Autodesk Inventor part; units mm, degrees
ref_plane "YZ Plane" through (0, 0, 0) normal (1, 0, 0) x (0, 1, 0)
ref_plane "XZ Plane" through (0, 0, 0) normal (0, 1, 0) x (-1, 0, 0)
ref_plane "XY Plane" through (0, 0, 0) normal (0, 0, 1) x (1, 0, 0)
sketch "Sketch1" plane through (0, 0, 0) normal (0, 0, 1) x (1, 0, 0)
  line L0 (-133.35, -63.5) -> (133.35, -63.5)
  line L1 (133.35, -63.5) -> (133.35, 63.5)
  line L2 (133.35, 63.5) -> (-133.35, 63.5)
  line L3 (-133.35, 63.5) -> (-133.35, -63.5)
  line L4 (-133.35, -63.5) -> (133.35, 63.5) construction
  line L5 (133.35, -63.5) -> (-133.35, 63.5) construction
  line L6 (0, 88.9) -> (0, -88.9) construction
  circle A0 centre (0, 47.625) radius 6.35
  circle A1 centre (-88.9, -47.625) radius 6.35
  circle A2 centre (88.9, -47.625) radius 6.35
  line L7 (-200.025, 0) -> (200.025, 0) construction
  point P0 (0, 0)
  point P1 (0, 0)
  dimension "d0" = 266.7
  dimension "d1" = 127
  dimension "d9" = 47.625
  dimension "d10" = 47.625
  dimension "d11" = 177.8
  dimension "d12" = 12.7
extrude "Extrusion2" add sketch "Sketch1" along normal blind 19.05
equation "\"d0\" = Length"
equation "\"d1\" = FrameHeight"
equation "\"d9\" = 0.375 * FrameHeight"
equation "\"d10\" = d9"
equation "\"d11\" = 0.666667 * Length"
equation "\"d7\" = Thickness"
equation "\"FrameHeight\" = 127"
properties part number "framePlate"
Read the model definition and answer for the solid it produces. Units are mm, in the model's axes. Coordinates: 2 decimals unless noted, no trailing zeros. Loops run counter-clockwise (first coordinate to the right, second up) from the corner with the lowest first, then second, coordinate; pieces in that order, holes last. Notation, with made-up numbers: (2, 13) - (16, 13) arc R26 ccw to (16, 48) - close; hole circle Ø7 at (45, 75). An arc over 180 degrees is marked (long way). Answer in a Markdown table with one row per item.
Q1. Find section A-A on x = 0. Write down the section's boundary in (y, z) (3 decimals), plus the area to 3 significant figures.
Here are the results:
| item | result |
|---|---|
| outline | (-63.5, 0) - (41.275, 0) - (41.275, 19.05) - (-63.5, 19.05) - close; (53.975, 0) - (63.5, 0) - (63.5, 19.05) - (53.975, 19.05) - close |
| area | 2,180 mm^2 |
Q2. The mould has two halves that part along Y. Classify faces 1 (the flat face through (-133.35, 1, 9)), 2 (the cylindrical face through (87.523, -41.426, 9.392)), 3 (the flat face through (-2, -63.5, 9)), 4 (the cylindrical face through (2.93, 53.26, 9.39)): pulls with the +Y half, pulls with the -Y half, needs draft (parallel to the pull), parting line crosses it, or undercut.
Here are the results:
| item | result |
|---|---|
| face 1 | needs draft |
| face 2 | undercut |
| face 3 | pulls with the -Y half |
| face 4 | undercut |
Q3. Given P1, Ø7.5, axis at x = -88.9, y = -47.625, coming from the -Z side, flat-ended and moving along its own axis, determine where the tip first touches the part or whether it passes through.
Here are the results:
| item | result |
|---|---|
| P1 | passes through |
Q4. Straight lines are drawn through the part: line 1 along X through (y, z) = (-43, 15); line 2 along Y through (x, z) = (-0.5, 8.75); line 3 along Y through (x, z) = (-88.9, 5) (3 decimals). For each, find the intervals that lie inside material, in ascending order. Write a range as [from, to].
Here are the results:
| item | result |
|---|---|
| line 1 | x = [-133.35, -93.25], [-84.55, 84.55], [93.25, 133.35] |
| line 2 | y = [-63.5, 41.29], [53.96, 63.5] |
| line 3 | y = [-63.5, -53.975], [-41.275, 63.5] |
